Source: CAD feature listing. Evaluate the final solid. Frame: model axes, mm. Face numbers are marked on the shaded views. A direction names the side the tool comes from. Give positions to 0.01 mm unless a question says otherwise; leave off trailing zeros. Order: outer loops, then holes, each group sorted by start corner. A loop starts at its lowest first (then second) coordinate and runs counter-clockwise, first axis right, second up. Notation, with made-up numbers: M -13.75,5.25 L 21.25,5.25 A17 cw 21.25,27.25 Z; hole C 47,41 d8. An arc over 180 degrees is marked long. One line per question, with ' | ' between items. Start each with the question number.
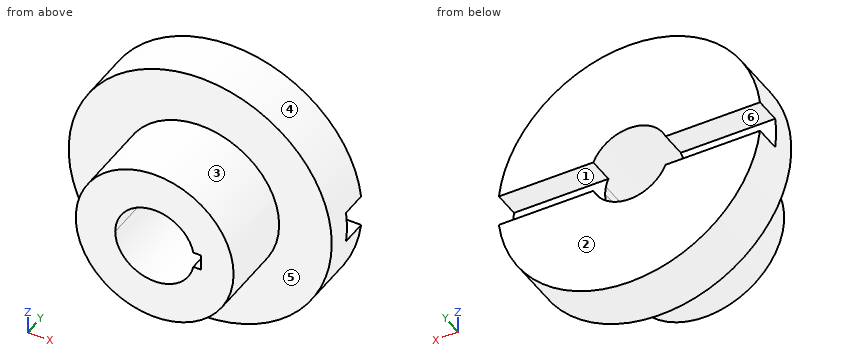
from build123d import *

# Parameters (mm, degrees)
F3_DEPTH = 50.001
F4_DEPTH = 30
F5_W     = 125.01227
F5_H     = 12
F6_DEPTH = 10


with BuildPart() as f1:
    # F0 (on Top) → F1 (revolve)
    with BuildSketch(Plane.XY):
        Polygon((0, 50), (0, 0), (30, 0), (30, 30), (50, 30), (50, 50), align=None)
    revolve(axis=Axis((0, 25, 0), (0, -1, 0)))

    # F2 (on face) → F3 (cut, through all)
    with BuildSketch(Plane.XZ):
        with BuildLine():
            Line((9.729625, 0), (15, 0))
            ThreePointArc((15, 0), (14.92405, 1.507558), (14.696969, 2.99985))
            Line((14.696969, 2.99985), (9.649316, 2.99985))
            Line((9.649316, 2.99985), (9.729625, 0))
        make_face()
        with BuildLine():
            ThreePointArc((-15, 0), (-1.507634, -14.924042), (14.696938, -3))
            Line((14.696938, -3), (9.809938, -3))
            Line((9.809938, -3), (9.729625, 0))
            Line((9.729625, 0), (-15, 0))
        make_face()
        with BuildLine():
            ThreePointArc((14.696938, -3), (14.924042, -1.507634), (15, 0))
            Line((15, 0), (9.729625, 0))
            Line((9.729625, 0), (9.809938, -3))
            Line((9.809938, -3), (14.696938, -3))
        make_face()
        with BuildLine():
            Line((9.649316, 2.99985), (14.696969, 2.99985))
            ThreePointArc((14.696969, 2.99985), (-1.507558, 14.92405), (-15, 0))
            Line((-15, 0), (9.729625, 0))
            Line((9.729625, 0), (9.649316, 2.99985))
        make_face()
    extrude(amount=-F3_DEPTH, mode=Mode.SUBTRACT)

    # F2 (on face) → F4 (cut)
    with BuildSketch(Plane.XZ):
        with BuildLine():
            Line((17.696969, 0), (15, 0))
            ThreePointArc((15, 0), (14.924042, -1.507634), (14.696938, -3))
            Line((14.696938, -3), (17.696969, -3))
            Line((17.696969, -3), (17.696969, 0))
        make_face()
        with BuildLine():
            ThreePointArc((14.696969, 2.99985), (14.92405, 1.507558), (15, 0))
            Line((15, 0), (17.696969, 0))
            Line((17.696969, 0), (17.696969, 2.99985))
            Line((17.696969, 2.99985), (14.696969, 2.99985))
        make_face()
        with BuildLine():
            Line((9.649316, 2.99985), (14.696969, 2.99985))
            ThreePointArc((14.696969, 2.99985), (-1.507558, 14.92405), (-15, 0))
            Line((-15, 0), (9.729625, 0))
            Line((9.729625, 0), (9.649316, 2.99985))
        make_face()
        with BuildLine():
            ThreePointArc((-15, 0), (-1.507634, -14.924042), (14.696938, -3))
            Line((14.696938, -3), (9.809938, -3))
            Line((9.809938, -3), (9.729625, 0))
            Line((9.729625, 0), (-15, 0))
        make_face()
    extrude(amount=-F4_DEPTH, mode=Mode.SUBTRACT)

    # F5 (on face) → F6 (cut)
    with BuildSketch(Plane(origin=(0, 50, 0), x_dir=(-1, 0, 0), z_dir=(0, 1, 0))):
        Rectangle(F5_W, F5_H)
    extrude(amount=-F6_DEPTH, mode=Mode.SUBTRACT)


solid = f1.part
Item 1: Cut plane A-A on y = 26. Return the cut outline in (x, z), and give its area (3 significant figures).
Item 2: Reachability of the marked faces 4, 5 and 6 from +Z, -Z, +X, -X, +Y, -Y: full face, straight path, thin tool, end or side. Return the list, or none.
Item 3: Cut plane B-B on z = 10.5. Return the cut outline in (x, y).
Item 4: Cut plane D-D on x = 19.5. Return the cut outline in (y, z).
Item 5: Mould query, pull axis Z, two halves, no side actions, for the marked faces 1, 2 and 3. Classes: pulls with the +Z half, pulls with the -Z half, needs draft (parallel to the pull), parting line crosses it, or undercut.
Item 6: Pin query (flat end, axial travel): pin 1 Ø5 at (y, z) = (12.5, -0.5) entering from -X; pin 2 Ø3.5 at (x, z) = (39.5, -0.5) entering from +Y; pin 3 Ø0.9 at (x, y) = (15.5, 14) entering from -Z; pin 4 Ø3.5 at (x, z) = (15.5, 1.5) entering from -Y. Return the tip coordinate at first contact, or that it passes through.
Item 7: Line query: line 1 (Y direction, x = -27.5, z = 4); line 2 (Y direction, x = -27, z = 29); line 3 (Z direction, x = -13, y = 34.5). Output: solid intervals per line, ascending.
Item 8: Cut plane C-C on x = -11.5. Return the cut outline in (y, z), and give its area (3 significant figures).
Results are:
1) outline: C 0,0 d60; hole M 14.7,-3 L 17.7,-3 L 17.7,3 L 14.7,3 A15 ccw long Z | area: 2,100 mm2
2) face 4: +Y, -Y | face 5: -Y | face 6: +X, -X, +Y
3) outline: M -48.89,30 L -28.1,30 L -28.1,0 L -10.71,0 L -10.71,50 L -48.89,50 Z; M 10.71,0 L 28.1,0 L 28.1,30 L 48.89,30 L 48.89,50 L 10.71,50 Z
4) outline: M 0,-22.8 L 30,-22.8 L 30,-46.04 L 50,-46.04 L 50,-6 L 40,-6 L 40,6 L 50,6 L 50,46.04 L 30,46.04 L 30,22.8 L 0,22.8 Z
5) face 1: undercut | face 2: needs draft | face 3: parting line crosses it
6) pin 1: stops at x = -30 | pin 2: stops at y = 40 | pin 3: stops at z = -25.95 | pin 4: stops at y = 0
7) line 1: y = 0 to 40 | line 2: y = 30 to 50 | line 3: z = -48.28 to -7.48, 7.48 to 48.28
8) outline: M 0,-27.71 L 30,-27.71 L 30,-48.66 L 50,-48.66 L 50,-9.63 L 0,-9.63 Z; M 0,9.63 L 50,9.63 L 50,48.66 L 30,48.66 L 30,27.71 L 0,27.71 Z | area: 2,650 mm2
